Design review of the part built by this model. Coordinates are the model's own, in mm. Face numbers are marked on the shaded views. A direction names the side the tool comes from. Round coordinates to 2 decimals unless told otherwise and drop trailing zeros. Loops run counter-clockwise (first coordinate to the right, second up) from the corner with the lowest first, then second, coordinate; pieces in that order, holes last. Notation, with made-up numbers: M 70.5,65.25 L 114.5,65.25 A12 cw 114.5,88.25 Z; hole C 31,8 d3. An arc over 180 degrees is marked long. One line per item, written item: value. Start each with the question number.
Item 1: We need section B-B (y = 1). Write out the cut boundary in (x, z).
Item 2: We need section D-D (y = -29.5). Write out the cut boundary in (x, z), then the cut area to 3 significant figures.
Item 3: We need section A-A (z = 15.75). Write out the cut boundary in (x, y), then the cut area to 3 significant figures.
Item 4: For the marked faces 1 and 2, list the 3-axis set-ups (+Z, -Z, +X, -X, +Y, -Y) from which the entire face can be reached by the end or side of a thin tool; tool diameter is ignored.
Item 5: Mouldability with a two-part tool opening along Y and no side actions: class the marked faces 3, 4 and 5 as released by +Y, released by -Y, zero draft, split by the parting line, or undercut.
Item 6: For line 1 along X through (y, z) = (17, 10.5); line 2 along Z through (x, y) = (4.5, 18.5); line 3 along X through (y, z) = (-30, 8.75), list the stretches that pass through material, from the lowest coordinate up.
Item 7: Clearance check with flat-ended pins moving along their axes: pin 1 (4 mm diameter, centred on x = 16, z = 3.5, fed in from -Y); pin 2 (2 mm diameter, centred on x = -12.5, z = 18, fed in from -Y); pin 3 (8 mm diameter, centred on x = 17, y = -31, fed in from -Z); pin 4 (2 mm diameter, centred on x = -1, y = 22, fed in from +Z). State where each tip first meets the part, or that it passes through.
Item 8: We need section C-C (x = 1). Write out the cut boundary in (y, z), then the cut area to 3 significant figures.
from build123d import *

# Parameters (mm, degrees)
F1_DEPTH = 25
F3_DEPTH = 2


with BuildPart() as f1:
    # F0 (on Top) → F1 (new body)
    with BuildSketch(Plane.XY):
        Polygon((-26, 31), (26, 31), (26, -13.102827), (10.982488, -31), (13.593303, -31), (28, -13.830767), (28, 33), (-28, 33), (-28, -13.830767), (-13.593303, -31), (-10.982488, -31), (-26, -13.102827), align=None)
    extrude(amount=F1_DEPTH)

    # F2 (on face) → F3 (join)
    with BuildSketch(Plane(origin=(0, 0, 0), x_dir=(1, 0, 0), z_dir=(0, 0, -1))):
        Polygon((-28, -33), (28, -33), (28, 13.830767), (12.006613, 33), (12.006613, 46.20152), (-11.915104, 46.20152), (-11.915104, 33), (-28, 13.830767), align=None)
    extrude(amount=F3_DEPTH)


solid = f1.part
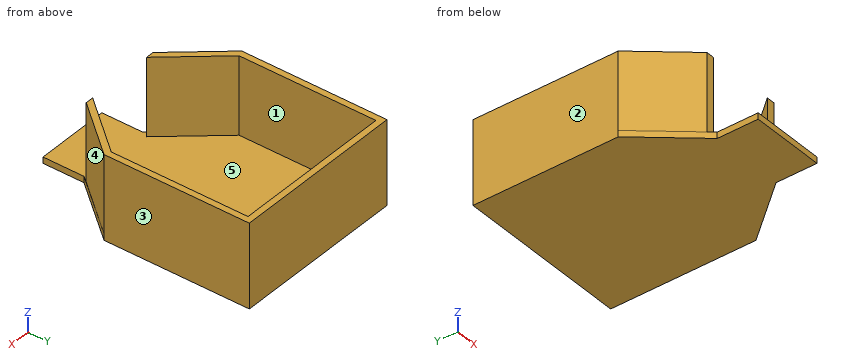
A:
1. outline: M -28,-2 L 28,-2 L 28,25 L 26,25 L 26,0 L -26,0 L -26,25 L -28,25 Z
2. outline: M -14.85,-2 L 14.93,-2 L 14.93,0 L 14.85,0 L 14.85,25 L 12.24,25 L 12.24,0 L -12.24,0 L -12.24,25 L -14.85,25 Z
2. area: 190 mm2
3. outline: M -28,-13.83 L -13.59,-31 L -10.98,-31 L -26,-13.1 L -26,31 L 26,31 L 26,-13.1 L 10.98,-31 L 13.59,-31 L 28,-13.83 L 28,33 L -28,33 Z
3. area: 381 mm2
4. face 1: +Z
4. face 2: +Z, -Z, -X, +Y, -Y
5. face 3: zero draft
5. face 4: released by -Y
5. face 5: undercut
6. line 1: -28 to -26, 26 to 28
6. line 2: -2 to 0
6. line 3: -14.43 to -11.82, 11.82 to 14.43
7. pin 1: y = -30.52
7. pin 2: y = -31
7. pin 3: z = -2
7. pin 4: z = 0
8. outline: M -46.2,-2 L 33,-2 L 33,25 L 31,25 L 31,0 L -46.2,0 Z
8. area: 208 mm2
